For this review, use the dimensioned drawing (mm, ordinates from the lowest corner) and the shaded views. A direction names the side the tool comes from. Coordinates: 2 decimals unless noted, no trailing zeros. Order: outer loops, then holes, each group sorted by start corner. A loop starts at its lowest first (then second) coordinate and runs counter-clockwise, first axis right, second up. Notation, with made-up numbers: M -14.75,12.25 L -4.75,12.25 A20 cw -4.75,49.25 Z; hole C -13.5,34 d3. An arc over 180 degrees is marked long. Answer in a Markdown table with one row per item.
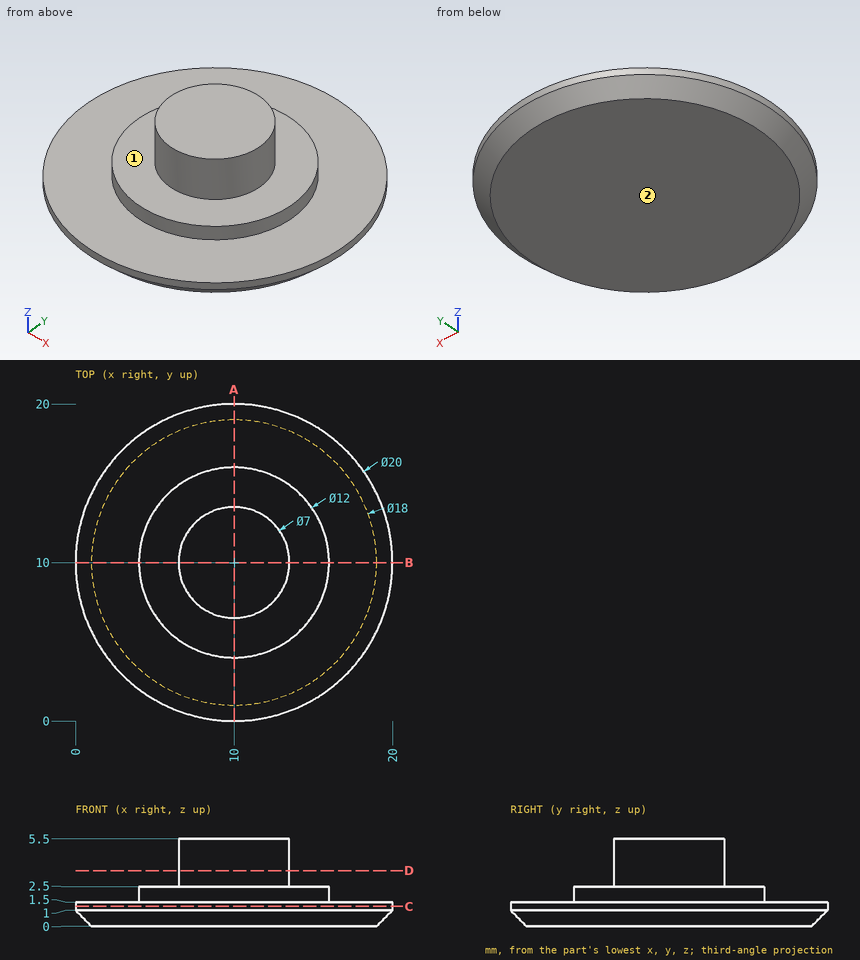
(1) For the marked faces 1 and 2, list the 3-axis set-ups (+Z, -Z, +X, -X, +Y, -Y) from which the entire face can be reached by the end or side of a thin tool; tool diameter is ignored.
Return value:
| item | result |
|---|---|
| face 1 | +Z |
| face 2 | -Z, +X, -X, +Y, -Y |
(2) For line 1 along Z through (x, y) = (11.5, 13.5); line 2 along Z through (x, y) = (4.75, 5.25); line 3 along Y through (x, z) = (10.25, 2.1), list the stretches that pass through material, from the lowest coordinate up. Write a range as from..to.
Return value:
| item | result |
|---|---|
| line 1 | z = 0..2.5 |
| line 2 | z = 0..1.5 |
| line 3 | y = 4.01..15.99 |
(3) Add section D-D, the plane z = 3.5. Give the boundary of the cut face in (x, y).
Return value:
| item | result |
|---|---|
| outline | C 10,10 d7 |
(4) Add section A-A, the plane x = 10. Give the boundary of the cut face in (y, z).
Return value:
| item | result |
|---|---|
| outline | M 0,1 L 1,0 L 19,0 L 20,1 L 20,1.5 L 16,1.5 L 16,2.5 L 13.5,2.5 L 13.5,5.5 L 6.5,5.5 L 6.5,2.5 L 4,2.5 L 4,1.5 L 0,1.5 Z |
(5) Insertion check: pin 1 Ø1.5 at (x, z) = (5, 3) entering from -Y; pin 2 Ø2 at (y, z) = (18, 4.5) entering from +X. Each pin has a flat end and moves straight along its axis. Give the tip position at first contact, or say it passes through.
Return value:
| item | result |
|---|---|
| pin 1 | stops at y = 5.97 |
| pin 2 | passes through |
(6) Add section C-C, the plane z = 1.25. Give the boundary of the cut face in (x, y), and give its area (3 significant figures).
Return value:
| item | result |
|---|---|
| outline | C 10,10 d20 |
| area | 314 mm2 |
